The listing builds one solid part. Answer for the finished solid, in the listing's coordinates (mm). A direction names the side the tool comes from. Give positions to 0.01 mm unless a question says otherwise; leave off trailing zeros. Order: outer loops, then holes, each group sorted by start corner. A loop starts at its lowest first (then second) coordinate and runs counter-clockwise, first axis right, second up. Notation, with made-up numbers: (-35.75, 4) - (-21.75, 4) arc R21 cw to (-21.75, 31) - close; hole circle Ø6 at (-38, 71.5). An arc over 180 degrees is marked (long way). Write each question's results on one line, items separated by ' | '. Start each with the question number.
1. Determine the mould class of faces 1 (the face through (-37, 35, -91)), 2 (the face through (-54.016, 37.676, 96.232)), 3 (the face through (-73, -27, -65)) for opening direction Z: released by +Z, released by -Z, zero draft, split by the parting line, or undercut.
2. Find the intervals of material crossed by L1, parallel to X at y = 11, z = 44; L2, parallel to X at y = 29, z = -18; L3, parallel to Z at x = -66, y = -15, in increasing order.
3. Section C-C (y = 47.5) is taken. Give the vertices of the cut face in (x, z).
4. Section D-D (y = 0) is taken. Give the vertices of the cut face in (x, z).
5. Section A-A (x = -41.5) is taken. Give the vertices of the cut face in (y, z), and give its area (3 significant figures).
6. Which of the six approach directions +Z, -Z, +X, -X, +Y, -Y give full straight-line access (tool end or side, diameter ignored) to faces 4 (the face through (-73, -25, 31)), 5 (the face through (-20.52, 37.33, -1.27)), 6 (the face through (-44, 18.5, 93))?
7. Section B-B (z = 41) is taken. Give the vertices of the cut face in (x, y), and give its area (3 significant figures).
8. Flat-ended cylindrical pins translate along their axes: pin 1 (6.5 mm diameter, centred on x = -74.5, z = 12.5, fed in from -Y); pin 2 (3 mm diameter, centred on y = 9, z = 93, fed in from +X); pin 3 (2 mm diameter, centred on x = -22.5, z = -59.5, fed in from -Y). Find the tip coordinate at first contact, or state that the pin passes through.
Autodesk Inventor part; units mm, degrees
ref_plane "Pracovní rovina2" through (-37.5, 0, 0) normal (1, 0, 0) x (0, 1, 0)
ref_plane "XZ Plane" through (0, 0, 0) normal (0, 1, 0) x (-1, 0, 0)
ref_plane "XY Plane" through (0, 0, 0) normal (0, 0, 1) x (1, 0, 0)
sketch "Náčrt1" plane through (0, 0, 0) normal (1, 0, 0) x (0, 1, 0)
  line L0 (25, 95) -> (-25, 95)
  line L1 (-25, 95) -> (-25, -95)
  line L2 (-25, -95) -> (25, -95)
  line L3 (25, -95) -> (25, 95)
  line L4 (25, 95) -> (-25, -95) construction
  line L5 (-25, 95) -> (25, -95) construction
  line L6 (-25, -3) -> (-29, -3)
  line L7 (-29, -3) -> (-29, 3)
  line L8 (-29, 3) -> (-25, 3)
  line L9 (-25, 3) -> (-25, -3)
  line L10 (-25, -65) -> (-29, -65)
  line L11 (-29, -65) -> (-29, -59)
  line L12 (-29, -59) -> (-25, -59)
  line L13 (-25, -59) -> (-25, -65)
  line L14 (-25, 59) -> (-29, 59)
  line L15 (-29, 59) -> (-29, 65)
  line L16 (-29, 65) -> (-25, 65)
  line L17 (-25, 65) -> (-25, 59)
  line L18 (7.5, 95) -> (7.5, 85)
  line L19 (7.5, 85) -> (17.5, 85)
  line L20 (17.5, 85) -> (17.5, 95)
  line L21 (-3.3333, 95) -> (-3.3333, 85)
  line L22 (-3.3333, 85) -> (-13.3333, 85)
  line L23 (-13.3333, 85) -> (-13.3333, 95)
  point P0 (0, 0)
  point P1 (25, 0)
  point P2 (-25, 0)
  point P3 (-25, 0)
  point P4 (-27, 3)
  point P5 (-27, 59)
  point P6 (12.5, 85)
  point P7 (-8.3333, 85)
  dimension "d0" = 50
  dimension "d1" = 190
  dimension "d46" = 6
  dimension "d47" = 4
  dimension "d48" = 4
  dimension "d49" = 6
  dimension "d50" = 30
  dimension "d51" = 4
  dimension "d52" = 6
  dimension "d53" = 30
  dimension "d54" = 56
  dimension "d73" = 10
  dimension "d74" = 10
  dimension "d75" = 10
  dimension "d76" = 10
  dimension "d77" = 12.5
  dimension "d78" = 16.6667
extrude "Vysunutí1" add sketch "Náčrt1" against normal blind 4
sketch "Náčrt2" plane through (0, 0, 0) normal (0, 0, 1) x (1, 0, 0)
  line L0 (-4, -25) -> (-4, 25)
  line L1 (4.3597, 25) -> (-37.5, 56.2403)
  line L2 (4.3597, 25) -> (-4, 25)
  line L3 (-4, 25) -> (-37.5, 50.0013)
  line L4 (-37.5, 56.2403) -> (-37.5, 50.0013)
  line L5 (0, -25) -> (0, 25)
  point P0 (0, 0)
  dimension "d56" = 31.2403
  dimension "d57" = 33.5
  dimension "d65" = 5
extrude "Vysunutí3" add sketch "Náčrt2" along normal mid plane 195
ref_plane "Pracovní rovina2" through (-37.5, 0, 0) normal (1, 0, 0) x (0, 1, 0)
mirror "Zrcadlit2" about plane through (-37.5, 0, 0) normal (1, 0, 0) of "Vysunutí3", "Vysunutí1"
sketch "Náčrt4" plane through (-4, -25, 95) normal (0, 0, 1) x (1, 0, 0)
  line L0 (4, 0) -> (0, 0)
  line L1 (-67, 50) -> (0, 50)
  line L2 (0, 50) -> (0, 0)
  line L3 (0, 0) -> (-67, 0)
  line L4 (-67, 0) -> (-67, 50)
  line L5 (-46, 43.5) -> (-21, 43.5)
  line L6 (-21, 43.5) -> (-21, 30.5)
  line L7 (-21, 30.5) -> (-46, 30.5)
  line L8 (-46, 30.5) -> (-46, 43.5)
  line L9 (-46, 43.5) -> (-21, 30.5) construction
  line L10 (-21, 43.5) -> (-46, 30.5) construction
  line L11 (-33, 43.5) -> (-33, 30.5)
  line L12 (-34, 43.5) -> (-34, 30.5)
  line L13 (-46, 37.5) -> (-21, 37.5)
  line L14 (-46, 36.5) -> (-21, 36.5)
  point P0 (4, 25)
  point P1 (-33.5, 37)
  point P2 (-33.5, 50)
  point P3 (-34, 36.5)
  point P4 (-33, 36.5)
  point P5 (-33, 37.5)
  point P6 (-34, 37.5)
  dimension "d30" = 50
  dimension "d31" = 67
  dimension "d34" = 25
  dimension "d35" = 13
  dimension "d37" = 21
  dimension "d38" = 1
  dimension "d39" = 1
  dimension "d41" = 6
  dimension "d42" = 12
  dimension "d43" = 25
  dimension "d66" = 6.5
extrude "Vysunutí5" add sketch "Náčrt4" against normal blind 4 contours L1 L2 L3 L4 | L5 L12 L13 L8 | L5 L11 L13 L12 | L13 L12 L14 L8 | L5 L6 L13 L11 | L13 L11 L14 L12 | L14 L12 L7 L8 | L13 L6 L14 L11 | L14 L11 L7 L12 | L14 L6 L7 L11
extrude "Vysunutí6" cut sketch "Náčrt4" against normal blind 10 contours L5 L12 L13 L8 | L5 L6 L13 L11 | L14 L12 L7 L8 | L14 L6 L7 L11
sketch "Náčrt5" plane through (0, -25, -95) normal (0, 0, -1) x (-1, 0, 0)
  line L0 (4, 50) -> (37.5, 75.0013)
  line L1 (4, 50) -> (71, 50)
  line L2 (4, 50) -> (37.5, 75.0013)
  line L3 (37.5, 75.0013) -> (71, 50)
  line L4 (37.5, 75.0013) -> (71, 50)
  line L5 (71, 50) -> (37.5, 75.0013)
  point P0 (0, 25)
  dimension "d67" = 67
extrude "Vysunutí7" add sketch "Náčrt5" against normal blind 4
mirror "Zrcadlit4" about plane through (0, 0, 0) normal (0, 0, 1) of "Vysunutí7"
sketch "Náčrt6" plane through (0, -25, 95) normal (0, 0, 1) x (1, 0, 0)
  line L0 (-75, 0) -> (0, 0)
  line L1 (-56.67, 0) -> (-56.67, -4)
  line L2 (-56.67, -4) -> (-50.67, -4)
  line L3 (-50.67, -4) -> (-50.67, 0)
  line L4 (-50.67, 0) -> (-56.67, 0)
  line L5 (-24.33, 0) -> (-24.33, -4)
  line L6 (-24.33, -4) -> (-18.33, -4)
  line L7 (-18.33, -4) -> (-18.33, 0)
  line L8 (-18.33, 0) -> (-24.33, 0)
  point P0 (0, 25)
  point P1 (-18.33, 0)
  point P2 (-24.33, 0)
  point P3 (-50.67, 0)
  dimension "d79" = 6
  dimension "d80" = 6
  dimension "d81" = 4
  dimension "d82" = 18.33
  dimension "d83" = 18.33
extrude "Vysunutí8" add sketch "Náčrt6" against normal blind 4
properties part number "prvni navrh"
Reported:
1) face 1: undercut | face 2: zero draft | face 3: released by -Z
2) L1: -75 to -71, -4 to 0 | L2: -74 to -65.64, -9.36 to -1 | L3: 91 to 95
3) outline: (-49.21, -97.5) - (-40.85, -97.5) - (-40.85, -95) - (-34.15, -95) - (-34.15, -97.5) - (-25.79, -97.5) - (-25.79, 97.5) - (-34.15, 97.5) - (-34.15, 95) - (-40.85, 95) - (-40.85, 97.5) - (-49.21, 97.5) - close; hole (-40.85, -91) - (-34.15, -91) - (-34.15, 91) - (-40.85, 91) - close
4) outline: (-75, -95) - (-71, -95) - (-71, 91) - (-4, 91) - (-4, -95) - (0, -95) - (0, 95) - (-75, 95) - close
5) outline: (-25, 91) - (5.5, 91) - (5.5, 95) - (-25, 95) - close; (11.5, 91) - (12.5, 91) - (12.5, 95) - (11.5, 95) - close; (18.5, 91) - (47.02, 91) - (47.02, -91) - (25, -91) - (25, -95) - (47.02, -95) - (47.02, -97.5) - (53.26, -97.5) - (53.26, 97.5) - (47.02, 97.5) - (47.02, 95) - (18.5, 95) - close | area: 1,540 mm²
6) face 4: +X, -X, -Y | face 5: -Y | face 6: +Z, -Z
7) outline: (-79.36, 25) - (-75, 25) - (-75, -25) - (-71, -25) - (-71, 25) - (-37.5, 50) - (-4, 25) - (-4, -25) - (0, -25) - (0, 25) - (4.36, 25) - (-37.5, 56.24) - close | area: 870 mm²
8) pin 1: y = -25 | pin 2: x = 0 | pin 3: y = 38.06
